from build123d import *

# Parameters (mm, degrees)
SKETCH1_R           = 15.875
BOSS_EXTRUDE1_DEPTH = 3.81
SKETCH2_R           = 9.144
BOSS_EXTRUDE2_DEPTH = 3.81
SKETCH3_W           = 9.525
SKETCH3_H           = 9.525
CUT_EXTRUDE1_DEPTH  = 9.652


with BuildPart() as part:
    # Sketch1 → Boss-Extrude1 (new body)
    with BuildSketch(Plane.XY):
        with Locations(Location((-130.201551665, 15.077630219, 0), (0, 0, 180))):
            Circle(SKETCH1_R)
    extrude(amount=BOSS_EXTRUDE1_DEPTH)

    # Sketch2 → Boss-Extrude2 (add)
    with BuildSketch(Plane(origin=(0, 0, 0), x_dir=(-1, 0, 0), z_dir=(0, 0, -1))):
        with Locations(Location((130.201551665, 15.077630219, 0), (0, 0, 180))):
            Circle(SKETCH2_R)
    extrude(amount=BOSS_EXTRUDE2_DEPTH)

    # Sketch3 → Cut-Extrude1 (cut)
    with BuildSketch(Plane(origin=(0, 0, -3.81), x_dir=(-1, 0, 0), z_dir=(0, 0, -1))):
        with Locations((130.201551665, 15.077630219)):
            Rectangle(SKETCH3_W, SKETCH3_H)
    extrude(amount=-CUT_EXTRUDE1_DEPTH, mode=Mode.SUBTRACT)


solid = part.part
Can you work these out from the model? Positions are in its coordinate system, mm. A direction names the side the tool comes from. Give positions to 0.01 mm unless a question says otherwise; leave off trailing zeros. Loops run counter-clockwise (first coordinate to the right, second up) from the corner with the lowest first, then second, coordinate; pieces in that order, holes last. Notation, with made-up numbers: M 71,-18 L 106,-18 A15 ccw 106,9 Z; hole C -16.75,-32 d5. An arc over 180 degrees is marked long. One line per item, written item: value. Start each with the question number.
1) If I drill on line 1 (Y direction, x = -130, z = -3); line 2 (Z direction, x = -119, y = 4); line 3 (Y direction, x = -132, z = 0.25), over which ranges is the centre line in solid material (lowest first)? Write a range as [from, to].
2) If we section it at B-B, the plane x = -126: Write out the boundary of the cut face in (y, z).
3) I'm going to push flat-ended pins straight in: pin 1 (1.5 mm diameter, centred on y = 24, z = 1.5, fed in from +X); pin 2 (4 mm diameter, centred on x = -128, z = -1, fed in from +Y). Where does each tip first touch, or does it pass through?
4) If we section it at D-D, the plane y = 6.5: Write out the boundary of the cut face in (x, z), and give its area (3 significant figures).
5) If we section it at A-A, the plane y = 18.5: Write out the boundary of the cut face in (x, z), and give its area (3 significant figures).
6) Thinking about a two-plate mould opening in Y: for faces 1 (the face through (-114.34, 14.38, 1.88)), 2 (the face through (-124, 15, -3.81)), 3 (the face through (-130, 10.315, 0)), which applies, +Y half, -Y half, draft (parallel to the pull), parting line (faces both ways), or undercut?
7) On a 3-axis mill with a long thin cutter (end or side, diameter ignored), from which of +Z, -Z, +X, -X, +Y, -Y can I reach the whole of each face in a straight line? I mean faces 4 (the face through (-137, 15, 3.81)), 5 (the face through (-125.439, 15, 0)), 6 (the face through (-139.337, 14.676, -1.878)). Say none if no direction works.
8) If we section it at C-C, the plane z = -2.25: Write out the boundary of the cut face in (x, y).
Completed:
1. line 1: y = [5.94, 10.32], [19.84, 24.22]
1. line 2: z = [0, 3.81]
1. line 3: y = [-0.7, 10.32], [19.84, 30.85]
2. outline: M -0.23,0 L 6.96,0 L 6.96,-3.81 L 10.32,-3.81 L 10.32,3.81 L -0.23,3.81 Z; M 19.84,-3.81 L 23.2,-3.81 L 23.2,0 L 30.39,0 L 30.39,3.81 L 19.84,3.81 Z
3. pin 1: stops at x = -116.59
3. pin 2: stops at y = 30.95
4. outline: M -143.56,0 L -133.37,0 L -133.37,-3.81 L -127.03,-3.81 L -127.03,0 L -116.84,0 L -116.84,3.81 L -143.56,3.81 Z
4. area: 126 mm^2
5. outline: M -145.7,0 L -138.68,0 L -138.68,-3.81 L -134.96,-3.81 L -134.96,3.81 L -145.7,3.81 Z; M -125.44,-3.81 L -121.72,-3.81 L -121.72,0 L -114.7,0 L -114.7,3.81 L -125.44,3.81 Z
5. area: 110 mm^2
6. face 1: parting line
6. face 2: draft
6. face 3: undercut
7. face 4: +Z, +X, -X, +Y, -Y
7. face 5: +Z, -Z
7. face 6: -Z
8. outline: C -130.2,15.08 d18.29; hole M -134.96,10.32 L -125.44,10.32 L -125.44,19.84 L -134.96,19.84 Z
